Here's how the part is built. I have some questions about the finished solid (model axes, mm). Face numbers are marked on the shaded views. A direction names the side the tool comes from. Give positions to 0.01 mm unless a question says otherwise; leave off trailing zeros. Write each loop counter-clockwise with the first axis right and the second up, starting at its lowest first coordinate (ties: lowest second). Pieces come first, ordered by that corner, then holes. Notation, with made-up numbers: (-32.5, 40) - (-24.5, 40) arc R13 cw to (-24.5, 58) - close; hole circle Ø10 at (-7.75, 16). An arc over 180 degrees is marked (long way). One line per item, written item: value. Start each with the question number.
1) I'm going to push flat-ended pins straight in: P1, Ø2, axis at y = 21, z = 5, coming from the +X side; P2, Ø0.8, axis at y = 19, z = -4, coming from the +X side; P3, Ø14, axis at y = 22.5, z = -28.5, coming from the +X side. Where does each tip first touch, or does it pass through?
2) Imagine slicing it at C-C on x = 10.25. Write out the boundary of the cut face in (y, z).
3) Please list where these lines run through material, in increasing order: L1, parallel to X at y = 3.25, z = -37; L2, parallel to X at y = 5.5, z = -31; L3, parallel to Z at x = 14.75, y = 32.5. Write a range as [from, to].
4) We'd pull the mould along Z, two halves only. Please class the marked faces 1, 2 and 3: +Z half, -Z half, draft (parallel to the pull), parting line (faces both ways), or undercut.
5) Imagine slicing it at B-B on y = 19. Count the separate pieces of the cut face and the enclosed holes in it, plus the area to 3 significant figures.
6) On a 3-axis mill with a long thin cutter (end or side, diameter ignored), from which of +Z, -Z, +X, -X, +Y, -Y can I reach the whole of each face in a straight line? I mean the marked faces 4, 5 and 6. Say none if no direction works.
7) Imagine slicing it at A-A on x = 14.75. Write out the boundary of the cut face in (y, z).
Autodesk Inventor part; units mm, degrees
ref_plane "YZ Plane" through (0, 0, 0) normal (1, 0, 0) x (0, 1, 0)
ref_plane "XZ Plane" through (0, 0, 0) normal (0, 1, 0) x (-1, 0, 0)
ref_plane "XY Plane" through (0, 0, 0) normal (0, 0, 1) x (1, 0, 0)
sketch "スケッチ1" plane through (0, 0, 0) normal (0, 1, 0) x (-1, 0, 0)
  line L0 (0, 0) -> (4, 0)
  line L1 (4, 0) -> (4, -40)
  line L2 (4, -40) -> (0, -40)
  line L3 (0, -40) -> (0, 0)
  line L4 (-3.5, 12.9904) -> (-6.9641, 10.9904)
  line L5 (-6.9641, 10.9904) -> (0.5359, -2)
  line L6 (0.5359, -2) -> (4, 0)
  line L7 (4, 0) -> (-3.5, 12.9904)
  line L8 (4, -40) -> (-23, -40)
  line L9 (-23, -40) -> (-23, -36)
  line L10 (-23, -36) -> (4, -36)
  line L11 (4, -36) -> (4, -40)
  line L12 (-3.5, 12.9904) -> (-1.5, 9.5263)
  line L13 (-1.5, 9.5263) -> (-24.8827, -3.9737)
  line L14 (-24.8827, -3.9737) -> (-26.8827, -0.5096)
  line L15 (-26.8827, -0.5096) -> (-3.5, 12.9904)
  line L16 (-23, -40) -> (-19, -40)
  line L17 (-19, -40) -> (-19, -7.2346)
  line L18 (-19, -7.2346) -> (-23, -7.2346)
  line L19 (-23, -7.2346) -> (-23, -40)
  line L20 (-26.8827, -0.5096) -> (-23.4186, 1.4904)
  line L21 (-23.4186, 1.4904) -> (-19.5359, -5.2346)
  line L22 (-19.5359, -5.2346) -> (-23, -7.2346)
  line L23 (-23, -7.2346) -> (-26.8827, -0.5096)
  line L24 (-23, -7.2346) -> (4, -7.2346)
  line L25 (4, -7.2346) -> (4, -11.2346)
  line L26 (4, -11.2346) -> (-23, -11.2346)
  line L27 (-23, -11.2346) -> (-23, -7.2346)
  line L28 (-19.5359, -5.2346) -> (-19, -7.2346)
  point P0 (0, -1.0718)
  point P1 (-21.4186, -1.9737)
  point P2 (-4.9641, 7.5263)
  point P3 (-24.8827, -3.9737)
  point P4 (0, -36)
  point P5 (-19, -36)
  point P6 (-19, -11.2346)
  point P7 (0, -11.2346)
  point P8 (0, -7.2346)
  dimension "d2" = 4
  dimension "d3" = 30
  dimension "d5" = 40
  dimension "d6" = 15
  dimension "d7" = 27
  dimension "d8" = 27
extrude "押し出し1" add sketch "スケッチ1" along normal blind 35 contours L3 L5 L13 L7 L0 | L0 L6 L5 L3 | L1 L24 L3 L5 L6 | L1 L26 L3 L24 | L13 L5 L4 L7 | L3 L26 L17 L24 | L13 L21 L15 L5 | L1 L10 L3 L26 | L17 L26 L19 L18 | L18 L22 L28 | L21 L22 L23 L13 | L13 L14 L15 L21 | L1 L2 L3 L10 | L3 L8 L17 L10 | L17 L10 L19 L26 | L17 L8 L9 L10
fillet "フィレット1" radius 8 4 edges at (-4, 17.5, 0) (23, 17.5, -7.2346) (19.5359, 17.5, -5.2346) (0, 17.5, -1.0718)
fillet "フィレット2" radius 3 12 edges at (3.5, 17.5, 12.9904) (26.8827, 17.5, -0.5096) (23, 17.5, -40) (-4, 17.5, -40) (0, 17.5, -11.2346) (19, 17.5, -36) (0, 17.5, -36) (19, 17.5, -11.2346) (4.9641, 17.5, 7.5263) (0, 17.5, -7.2346) (19, 17.5, -7.2346) (21.4186, 17.5, -1.9737)
sketch "スケッチ2" plane through (0, 35, 0) normal (0, 1, 0) x (1, 0, 0)
  circle A0 centre (4.5981, -8.8923) radius 1
  arc A1 (2, -10.3923) -> (6.0981, -11.4904) centre (4.5981, -8.8923) ccw
  circle A2 centre (22.7846, 1.6077) radius 1
  circle A3 centre (20, 37) radius 1
  circle A4 centre (20, 9.2346) radius 1
  circle A5 centre (-1, 9.2346) radius 1
  circle A6 centre (-1, 37) radius 1
  arc A7 (24.2846, -0.9904) -> (25.3827, 3.1077) centre (22.7846, 1.6077) ccw
  arc A8 (-1, 40) -> (-4, 37) centre (-1, 37) ccw
  arc A9 (23, 37) -> (20, 40) centre (20, 37) ccw
  line L0 (3, 7.2346) -> (16.7785, 7.2346)
  line L1 (16, 11.2346) -> (3, 11.2346)
  point P0 (0, 0)
  dimension "d10" = 2
  dimension "d11" = 2
  dimension "d12" = 2
  dimension "d13" = 2
  dimension "d14" = 2
  dimension "d15" = 2
  dimension "d16" = 2
  dimension "d17" = 2
extrude "押し出し2" cut sketch "スケッチ2" against normal through all
sketch "スケッチ3" plane through (24.0718, 0, -5.3782) normal (0.866, 0, -0.5) x (-0.5, 0, -0.866)
  line L0 (-2.6218, 0) -> (-2.6218, 35)
  line L1 (-2.6218, 0) -> (0, 0)
  line L2 (0, 35) -> (0, 0)
  line L3 (-2.6218, 35) -> (0, 35)
  line L4 (0, 12.5) -> (-14.5476, 12.5)
  line L5 (-14.5476, 12.5) -> (-14.5476, 22.5)
  line L6 (-14.5476, 22.5) -> (0, 22.5)
  line L7 (0, 22.5) -> (0, 12.5)
  line L8 (0, 35) -> (0, 0)
  point P0 (7.3782, 0)
  point P1 (0, 17.5)
  point P2 (0, 17.5)
  dimension "d20" = 10
extrude "押し出し3" cut sketch "スケッチ3" against normal blind 10 contours L4 L5 L6 L0 | L0 L6 L2 L4
sketch "スケッチ5" plane through (16, 0, -11.2346) normal (0, 0, -1) x (-1, 0, 0)
  line L0 (0, 0) -> (0, 35)
  line L1 (0, 0) -> (13, 0)
  line L2 (13, 35) -> (13, 0)
  line L3 (0, 35) -> (13, 35)
  line L4 (0, 35) -> (13, 35)
  line L5 (13, 35) -> (0, 0)
  line L6 (13, 0) -> (0, 35)
  circle A0 centre (6.5, 17.5) radius 6
  point P0 (16, 0)
  dimension "d26" = 12
extrude "押し出し5" cut sketch "スケッチ5" against normal up to surface (4 mm away) contours A0 L6 L5 | L5 L6 A0 | A0 L5 L6 | L6 L5 A0
sketch "スケッチ6" plane through (20, 0, -40) normal (0, 0, -1) x (-1, 0, 0)
  line L0 (21, 35) -> (21, 0)
  line L1 (0, 35) -> (21, 35)
  line L2 (0, 0) -> (0, 35)
  line L3 (0, 0) -> (21, 0)
  line L4 (10.5, 25) -> (-9.5, 25)
  line L5 (-9.5, 25) -> (-9.5, 10)
  line L6 (-9.5, 10) -> (10.5, 10)
  line L7 (10.5, 10) -> (10.5, 25)
  line L8 (0, 0) -> (21, 0)
  line L9 (21, 35) -> (21, 0)
  point P0 (20, 0)
  point P1 (10.5, 0)
  point P2 (10.5, 17.5)
  point P3 (21, 17.5)
  dimension "d29" = 15
extrude "押し出し6" cut sketch "スケッチ6" against normal blind 10 contours L4 L7 L6 L2 | L2 L6 L5 L4
equation "\"d16\" = d17"
properties part number "leg_upper_middle"
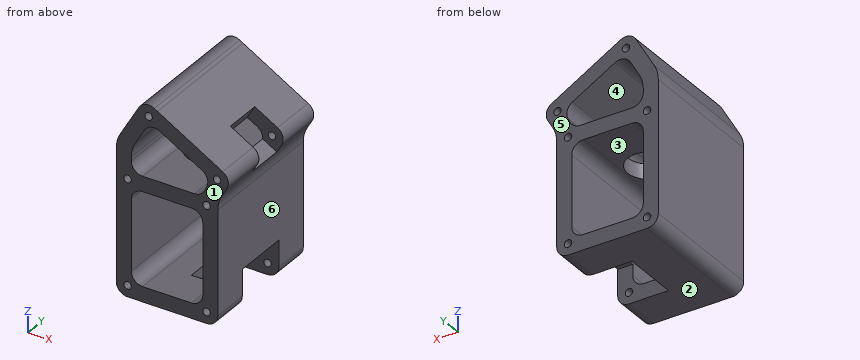
Numbers:
1. P1: x = 18.22
1. P2: x = 22.38
1. P3: x = 23
2. outline: (0, -40) - (10, -40) - (10, -36) - (0, -36) - close; (0, -11.23) - (11.55, -11.23) - (11.55, -7.23) - (0, -7.23) - close; (0, 4.47) - (35, 4.47) - (35, 9.09) - (0, 9.09) - close; (23.45, -11.23) - (35, -11.23) - (35, -7.23) - (23.45, -7.23) - close; (25, -40) - (35, -40) - (35, -36) - (25, -36) - close
3. L1: [-4, -2], [0, 19], [21, 23]
3. L2: [-4, 0], [19, 23]
3. L3: [-40, -36], [-11.23, -7.23], [1.88, 6.5]
4. face 1: draft
4. face 2: -Z half
4. face 3: undercut
5. separate pieces: 2
5. enclosed holes: 4
5. area: 433 mm^2
6. face 4: +Y, -Y
6. face 5: +Z, -Z, +X, -X, +Y
6. face 6: -Z, +X, +Y, -Y
7. outline: (0, -40) - (10, -40) - (10, -36) - (0, -36) - close; (0, -11.23) - (14.6, -11.23) - (14.6, -7.23) - (0, -7.23) - close; (0, 1.88) - (35, 1.88) - (35, 6.5) - (0, 6.5) - close; (20.4, -11.23) - (35, -11.23) - (35, -7.23) - (20.4, -7.23) - close; (25, -40) - (35, -40) - (35, -36) - (25, -36) - close
